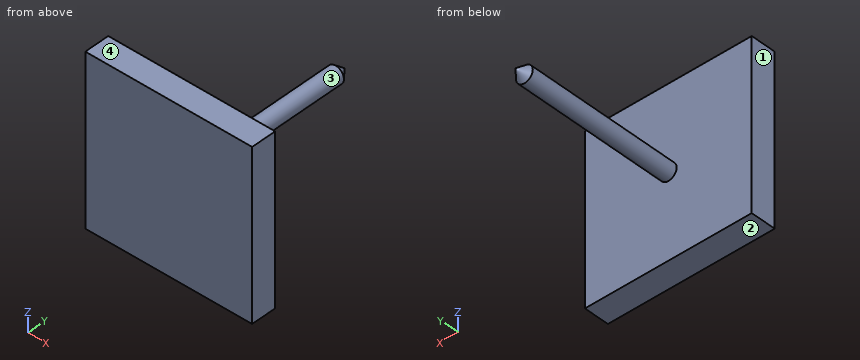
```python
from build123d import *

# Parameters (mm, degrees)
CROQUIS1_W              = 20
CROQUIS1_H              = 20
SALIENTE_EXTRUIR1_DEPTH = 3


with BuildPart() as part:
    # Croquis1 → Saliente-Extruir1 (new body)
    with BuildSketch(Plane(origin=(0, 0, 0), x_dir=(1, 0, 0), z_dir=(0, 1, 0))):
        with Locations((10, 10)):
            Rectangle(CROQUIS1_W, CROQUIS1_H)
    extrude(amount=SALIENTE_EXTRUIR1_DEPTH)

    # Croquis2 → Revolución1 (revolve)
    with BuildSketch(Plane(origin=(10, 0, 0), x_dir=(0, 0, -1), z_dir=(1, 0, 0))):
        Polygon((10, 3), (10, 23), (11, 21.808246407), (11, 3), align=None)
    revolve(axis=Axis((10, 3, -10), (0, 1, 0)))


solid = part.part
```
CAD build for the part. Positions are in the model's coordinates, mm. Face numbers are marked on the shaded views. Round coordinates to 2 decimals unless told otherwise and drop trailing zeros. Order: outer loops, then holes, each group sorted by start corner. A loop starts at its lowest first (then second) coordinate and runs counter-clockwise, first axis right, second up.
Q1. Drop flat-ended pins along their axis: pin 1 (10 mm diameter, centred on x = 10.5, y = 19.5, fed in from -Z); pin 2 (10 mm diameter, centred on y = 20.5, z = -2, fed in from +X); pin 3 (8 mm diameter, centred on x = 15.5, z = -6, fed in from +Y). Give the stop position or say it passes through.
Q2. Two-plate mould, pull along Z, no slides. Class the marked faces 1, 2, 3 and 4: pulls with the +Z half, pulls with the -Z half, needs draft (parallel to the pull), parting line crosses it, or undercut.
Q3. Slice it at B-B (y = 13.25). Write the cut outline in (x, z).
Q4. Slice it at C-C (z = -7.25). Write the cut outline in (x, y), and give its area (3 significant figures).
Q5. Slice it at A-A (x = 8). Write the cut outline in (y, z).
Q6. Wall check: L1, parallel to Z at x = 10, y = 7; L2, parallel to Y at x = 11.75, z = -2.5; L3, parallel to X at y = 13.5, z = -10.75. Give the ranges that are in metal, low to high.
Results below:
1. pin 1: stops at z = -11
1. pin 2: passes through
1. pin 3: stops at y = 3
2. face 1: needs draft
2. face 2: pulls with the -Z half
2. face 3: parting line crosses it
2. face 4: pulls with the +Z half
3. outline: circle Ø2 at (10, -10)
4. outline: (0, 0) - (20, 0) - (20, 3) - (0, 3) - close
4. area: 60.0 mm2
5. outline: (0, -20) - (3, -20) - (3, 0) - (0, 0) - close
6. L1: z = -11 to -9
6. L2: y = 0 to 3
6. L3: x = 9.34 to 10.66
